Geometry check sheet. Reference: the model listing, model coordinates, mm. A direction names the side the tool comes from. Round coordinates to 2 decimals unless told otherwise and drop trailing zeros.
Autodesk Inventor part; units mm, degrees
ref_plane "YZ Plane" through (0, 0, 0) normal (1, 0, 0) x (0, 1, 0)
ref_plane "XZ Plane" through (0, 0, 0) normal (0, 1, 0) x (-1, 0, 0)
ref_plane "XY Plane" through (0, 0, 0) normal (0, 0, 1) x (1, 0, 0)
sketch "Block1" plane through (0, 0, 0) normal (0, 0, 1) x (1, 0, 0)
  circle A0 centre (250, 0) radius 40 construction
  arc A1 (284, 0) -> (274.0416, -24.0416) centre (250, 0) ccw construction
  circle A2 centre (250, 0) radius 10.05 construction
  arc A3 (276, 0) -> (268.3848, -18.3848) centre (250, 0) ccw construction
  circle A4 centre (280, 0) radius 1.6 construction
  arc A5 (276, 0) -> (284, 0) centre (280, 0) ccw construction
  circle A6 centre (271.2132, -21.2132) radius 1.6 construction
  arc A7 (274.0416, -24.0416) -> (268.3848, -18.3848) centre (271.2132, -21.2132) ccw construction
  point P0 (269.205, -7.955)
  dimension "d0" = 8
sketch "Sketch1" plane through (0, 0, 0) normal (0, 0, 1) x (1, 0, 0)
  arc A0 (18.4908, -18.4908) -> (0, -26.15) centre (0, 0) ccw
  arc A1 (23.9356, -23.9356) -> (0, -33.85) centre (0, 0) ccw
  arc A2 (0, -33.85) -> (0, -26.15) centre (0, -30) ccw
  circle A3 centre (0, -30) radius 2.9
  arc A4 (18.4908, -18.4908) -> (23.9356, -23.9356) centre (21.2132, -21.2132) ccw
  circle A5 centre (21.2132, -21.2132) radius 2.9
  circle A6 centre (30, 0) radius 2.9
  circle A7 centre (21.2132, 21.2132) radius 2.9
  circle A8 centre (0, 30) radius 2.9
  circle A9 centre (-21.2132, 21.2132) radius 2.9
  circle A10 centre (-30, 0) radius 2.9
  circle A11 centre (-21.2132, -21.2132) radius 2.9
  point P0 (0, 0)
  point P1 (0, 0)
  dimension "d1" = 0.15
  dimension "d2" = 5.8
  dimension "d5" = 360
extrude "Extrusion1" add sketch "Sketch1" along normal blind 2
sketch "Sketch2" plane through (0, 0, 2) normal (0, 0, 1) x (1, 0, 0)
  arc A0 (23.9356, -23.9356) -> (0, -33.85) centre (0, 0) ccw
  arc A1 (0, -33.85) -> (0, -26.15) centre (0, -30) ccw
  arc A2 (18.4908, -18.4908) -> (0, -26.15) centre (0, 0) ccw
  arc A3 (18.4908, -18.4908) -> (23.9356, -23.9356) centre (21.2132, -21.2132) ccw
  circle A4 centre (0, 30) radius 2.9
  circle A5 centre (30, 0) radius 2.9
  circle A6 centre (21.2132, -21.2132) radius 2.9
  circle A7 centre (-30, 0) radius 2.9
  circle A8 centre (-21.2132, -21.2132) radius 2.9
  circle A9 centre (-21.2132, 21.2132) radius 2.9
  circle A10 centre (21.2132, 21.2132) radius 2.9
  circle A11 centre (0, -30) radius 2.9
  point P0 (0, 0)
extrude "Extrusion2" add sketch "Sketch2" along normal blind 0.6 contours A3 A2 A1 A0 | A4 | A5 | A6 | A7 | A8 | A9 | A10 | A11
fillet "Fillet1" radius 1 4 edges at (3.85, -30, 2.6) (-10.0072, 24.1594, 2.6) (18.4908, -23.9356, 2.6) (-12.9538, 31.2733, 2.6)
properties part number "LogoCover"
1) Scan lines: line 1 along Y through (x, z) = (0, 1); line 2 along Y through (x, z) = (20, 1.25); line 3 along X through (y, z) = (-6, 2.3). Record each from-to range of solid material in increasing order.
Report:
line 1: y = -33.85 to -32.9, -27.1 to -26.15, 26.15 to 27.1, 32.9 to 33.85
line 2: y = -24.87 to -23.85, -18.58 to -16.85, 16.85 to 18.58, 23.85 to 27.31
line 3: x = -33.02 to -25.75, 25.75 to 33.02
2) Gauge pin test, flat end, axial feed: pin 1 (3 mm diameter, centred on x = -21.5, y = -21.5, fed in from -Z). Record the tip position at first contact, or that the pin passes through.
Report:
pin 1: stops at z = 2
3) Sectioned sample at A-A, the plane z = 0.75. State how many separate pieces and enclosed holes the cut face has, then the cut area to 3 significant figures.
Report:
separate pieces: 1
enclosed holes: 8
area: 1,110 mm2
4) Access from +Z, -Z, +X, -X, +Y, -Y to the whole of each face (thin tool, end or side, straight path). Record for faces 4 (the face through (21, -21, 2)), 5 (the face through (3.85, -29.92, 0.79)).
Report:
face 4: -Z
face 5: +Z, -Z, +X
5) Mould release check, pull along Y, two halves, no side actions. Record for faces 1 (the face through (-30, 0, 2)), 2 (the face through (-7.7, 25.2, 0)), 3 (the face through (-14.15, 30.75, 0.79)): +Y half, -Y half, draft (parallel to the pull), parting line (faces both ways), or undercut.
Report:
face 1: undercut
face 2: draft
face 3: parting line
